from build123d import *

# Parameters (mm, degrees)
SKETCH5_W           = 395.4
SKETCH5_H           = 265.4
BOSS_EXTRUDE3_DEPTH = 6.35
SKETCH6_W           = 78.175
SKETCH6_H           = 243.175
SKETCH6_W_2         = 75
SKETCH6_H_2         = 240
CUT_EXTRUDE1_DEPTH  = 6.35
SKETCH10_W          = 6.35
SKETCH10_H          = 50.8
SKETCH10_W_2        = 50.8
SKETCH10_H_2        = 6.35
CUT_EXTRUDE2_DEPTH  = 6.35
SKETCH11_W          = 50.8
SKETCH11_H          = 6.35
CUT_EXTRUDE3_DEPTH  = 6.35
SKETCH12_W          = 78.175
SKETCH12_H          = 4.7625
BOSS_EXTRUDE4_DEPTH = 6.35
FILLET1_R           = 3.175
CUT_EXTRUDE4_DEPTH  = 239.190895082


with BuildPart() as part:
    # Sketch5 → Boss-Extrude3 (new body)
    with BuildSketch(Plane(origin=(0, 0, 0), x_dir=(1, 0, 0), z_dir=(0, 1, 0))):
        Rectangle(SKETCH5_W, SKETCH5_H)
    extrude(amount=BOSS_EXTRUDE3_DEPTH)

    # Sketch6 → Cut-Extrude1 (cut)
    # profile 1 of 4: a face of its own
    with BuildSketch(Plane(origin=(0, 6.35, 0), x_dir=(1, 0, 0), z_dir=(0, 1, 0))):
        with Locations((147.5, 0)):
            Rectangle(SKETCH6_W, SKETCH6_H)
        with Locations((147.5, 0)):
            Rectangle(SKETCH6_W_2, SKETCH6_H_2, mode=Mode.SUBTRACT)
    # profile 2 of 4: a face of its own
    with BuildSketch(Plane(origin=(0, 6.35, 0), x_dir=(1, 0, 0), z_dir=(0, 1, 0))):
        with Locations((147.5, 0)):
            Rectangle(SKETCH6_W_2, SKETCH6_H_2)
    # profile 3 of 4: a face of its own
    with BuildSketch(Plane(origin=(0, 6.35, 0), x_dir=(1, 0, 0), z_dir=(0, 1, 0))):
        with Locations((-147.5, 0)):
            Rectangle(SKETCH6_W, SKETCH6_H)
        with Locations((-147.5, 0)):
            Rectangle(SKETCH6_W_2, SKETCH6_H_2, mode=Mode.SUBTRACT)
    # profile 4 of 4: a face of its own
    with BuildSketch(Plane(origin=(0, 6.35, 0), x_dir=(1, 0, 0), z_dir=(0, 1, 0))):
        with Locations((-147.5, 0)):
            Rectangle(SKETCH6_W_2, SKETCH6_H_2)
    extrude(amount=-CUT_EXTRUDE1_DEPTH, mode=Mode.SUBTRACT)

    # Sketch10 → Cut-Extrude2 (cut)
    with BuildSketch(Plane.XZ):
        with Locations((98.8875, -63.5)):
            Rectangle(SKETCH10_W, SKETCH10_H)
        with Locations((98.8875, 63.5)):
            Rectangle(SKETCH10_W, SKETCH10_H)
        with Locations((-98.8875, 63.5)):
            Rectangle(SKETCH10_W, SKETCH10_H)
        with Locations((-98.8875, -63.5)):
            Rectangle(SKETCH10_W, SKETCH10_H)
        Polygon((197.7, 132.7), (177.8, 132.7), (177.8, 126.35), (191.35, 126.35), (197.7, 126.35), align=None)
        Polygon((127, 132.7), (76.2, 132.7), (76.2, 126.35), (95.7125, 126.35), (102.0625, 126.35), (108.4125, 126.35), (127, 126.35), align=None)
        with Locations((0, 129.525)):
            Rectangle(SKETCH10_W_2, SKETCH10_H_2)
        Polygon((-127, 132.7), (-127, 126.35), (-108.4125, 126.35), (-102.0625, 126.35), (-95.7125, 126.35), (-76.2, 126.35), (-76.2, 132.7), align=None)
        Polygon((-197.7, 126.35), (-191.35, 126.35), (-177.8, 126.35), (-177.8, 132.7), (-197.7, 132.7), align=None)
        Polygon((-177.8, -126.35), (-191.35, -126.35), (-197.7, -126.35), (-197.7, -132.7), (-177.8, -132.7), align=None)
        Polygon((-108.4125, -126.35), (-127, -126.35), (-127, -132.7), (-76.2, -132.7), (-76.2, -126.35), (-95.7125, -126.35), (-102.0625, -126.35), align=None)
        with Locations((0, -129.525)):
            Rectangle(SKETCH10_W_2, SKETCH10_H_2)
        Polygon((76.2, -126.35), (76.2, -132.7), (127, -132.7), (127, -126.35), (108.4125, -126.35), (102.0625, -126.35), (95.7125, -126.35), align=None)
        Polygon((177.8, -126.35), (177.8, -132.7), (197.7, -132.7), (197.7, -126.35), (191.35, -126.35), align=None)
    extrude(amount=-CUT_EXTRUDE2_DEPTH, mode=Mode.SUBTRACT)

    # Sketch11 → Cut-Extrude3 (cut)
    with BuildSketch(Plane(origin=(197.7, 0, 0), x_dir=(0, 0, -1), z_dir=(1, 0, 0))):
        with Locations((-63.5, 3.175)):
            Rectangle(SKETCH11_W, SKETCH11_H)
        with Locations((63.5, 3.175)):
            Rectangle(SKETCH11_W, SKETCH11_H)
    cut_extrude3 = extrude(amount=-CUT_EXTRUDE3_DEPTH, mode=Mode.SUBTRACT)

    # Mirror1: Cut-Extrude3 across plane
    add(cut_extrude3.mirror(Plane(origin=(0, 0, 0), x_dir=(0, 0, 1), z_dir=(1, 0, 0))), mode=Mode.SUBTRACT)

    # Sketch12 → Boss-Extrude4 (add)
    with BuildSketch(Plane.XZ):
        with Locations((147.5, -119.20625)):
            Rectangle(SKETCH12_W, SKETCH12_H)
        with Locations((147.5, 119.20625)):
            Rectangle(SKETCH12_W, SKETCH12_H)
        with Locations((-147.5, 119.20625)):
            Rectangle(SKETCH12_W, SKETCH12_H)
        with Locations((-147.5, -119.20625)):
            Rectangle(SKETCH12_W, SKETCH12_H)
    extrude(amount=-BOSS_EXTRUDE4_DEPTH)

    # Fillet1
    fillet1_edges = [part.edges().sort_by_distance(p)[0] for p in [
        (108.4125, 3.175, -116.825),
        (186.5875, 3.175, -116.825),
        (186.5875, 3.175, 116.825),
        (108.4125, 3.175, 116.825),
        (-186.5875, 3.175, 116.825),
        (-108.4125, 3.175, 116.825),
        (-108.4125, 3.175, -116.825),
        (-186.5875, 3.175, -116.825),
    ]]
    fillet(fillet1_edges, radius=FILLET1_R)

    # Sketch13 → Cut-Extrude4 (cut, through all)
    with BuildSketch(Plane.XZ):
        Polygon((25.4, -132.7), (69.85, -132.7), (69.85, 132.7), (25.4, 132.7), (25.4, 126.35), (-25.4, 126.35), (-25.4, 132.7), (-69.85, 132.7), (-69.85, -132.7), (-25.4, -132.7), (-25.4, -126.35), (25.4, -126.35), align=None)
        Polygon((-76.2, -132.7), (-69.85, -132.7), (-69.85, 132.7), (-76.2, 132.7), (-76.2, 126.35), (-127, 126.35), (-127, 132.7), (-177.8, 132.7), (-177.8, 126.35), (-197.7, 126.35), (-197.7, 88.9), (-191.35, 88.9), (-191.35, 38.1), (-197.7, 38.1), (-197.7, -38.1), (-191.35, -38.1), (-191.35, -88.9), (-197.7, -88.9), (-197.7, -126.35), (-177.8, -126.35), (-177.8, -132.7), (-127, -132.7), (-127, -126.35), (-76.2, -126.35), align=None)
    extrude(amount=-CUT_EXTRUDE4_DEPTH, mode=Mode.SUBTRACT)


solid = part.part
Geometry: final body of the model. Coordinates: model frame, mm. A direction names the side the tool comes from. Coordinates: 2 decimals unless noted, no trailing zeros. Loops run counter-clockwise (first coordinate to the right, second up) from the corner with the lowest first, then second, coordinate; pieces in that order, holes last. Notation, with made-up numbers: (29.25, 1.25) - (76.25, 1.25) arc R28 cw to (76.25, 40.25) - close; hole circle Ø1 at (-3, 69). An arc over 180 degrees is marked (long way). One line per question, with ' | ' between items. Start each with the question number.
(1) Ray query, L1, parallel to X at y = 3.5, z = 51; L2, parallel to X at y = 4.25, z = -109; L3, parallel to Z at x = 162, y = 5.5 (3 decimals). Return the intervals inside material, ascending. Write a range as from..to.
(2) Cut plane A-A on x = 119.5. Output: boundary loops of the cut face in (y, z) (3 decimals).
(3) First-contact query: pin 1 (1.9 mm diameter, centred on y = 3.5, z = 130, fed in from +X); pin 2 (3 mm diameter, centred on x = 110.5, z = -49, fed in from -Y); pin 3 (1.9 mm diameter, centred on x = 194.5, y = 4, fed in from +Z). Flat tips, straight axial feed; report the tip coordinate or a pass-through.
(4) Cut plane C-C on z = -66. Output: boundary loops of the cut face in (x, y), and give its area (3 significant figures).
(5) Cut plane B-B on z = -97.5. Output: boundary loops of the cut face in (x, y).
(6) Cut plane D-D on y = 1.75. Count the separate pieces of the cut face and the enclosed holes in it, and give its area (3 significant figures).
(7) Reachability of faces 1 (the flat face through (102, 3, -126.35)), 2 (the flat face through (76.2, 3, 130)), 3 (the flat face through (195, 3, 88.9)) from +Z, -Z, +X, -X, +Y, -Y: full face, straight path, thin tool, end or side. Return the list, or none.
(8) Draft query along X for faces 4 (the flat face through (177.8, 3, -129)), 5 (the flat face through (102.062, 3, 63)), 6 (the flat face through (152, 3, 132.7)). Return one class per face: +X half, -X half, draft (parallel to the pull), parting line (faces both ways), or undercut.
Here are the results:
1) L1: 69.85..95.71, 102.06..108.41, 186.59..191.35 | L2: 69.85..108.41, 186.59..197.7 | L3: -132.7..-116.825, 116.825..132.7
2) outline: (0, -126.35) - (6.35, -126.35) - (6.35, -116.825) - (0, -116.825) - close; (0, 116.825) - (6.35, 116.825) - (6.35, 126.35) - (0, 126.35) - close
3) pin 1: x = 177.8 | pin 2: through | pin 3: z = 126.35
4) outline: (69.85, 0) - (95.71, 0) - (95.71, 6.35) - (69.85, 6.35) - close; (102.06, 0) - (108.41, 0) - (108.41, 6.35) - (102.06, 6.35) - close; (186.59, 0) - (191.35, 0) - (191.35, 6.35) - (186.59, 6.35) - close | area: 235 mm²
5) outline: (69.85, 0) - (108.41, 0) - (108.41, 6.35) - (69.85, 6.35) - close; (186.59, 0) - (197.7, 0) - (197.7, 6.35) - (186.59, 6.35) - close
6) separate pieces: 1 | enclosed holes: 3 | area: 13,500 mm²
7) face 1: -Z, +Y, -Y | face 2: +Z, +Y, -Y | face 3: +X, +Y, -Y
8) face 4: +X half | face 5: undercut | face 6: draft
